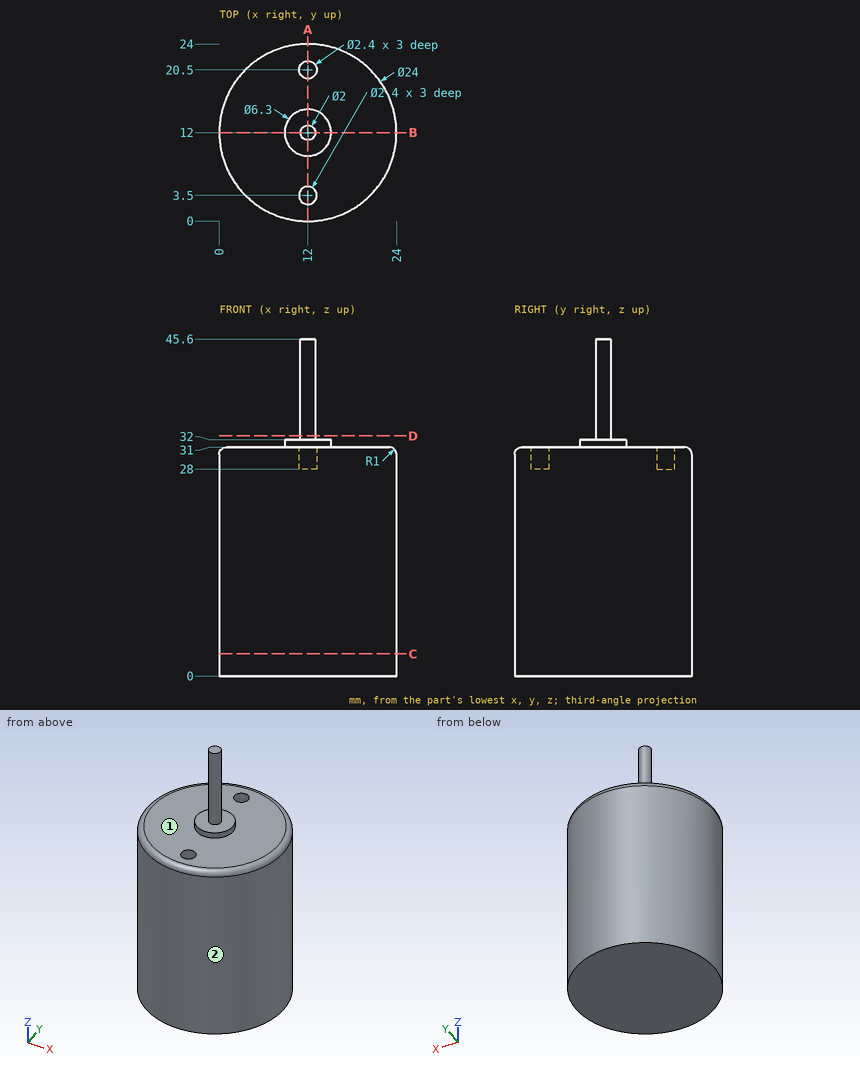
The figure shows three views and two pictorial views of one solid part (mm, origin at its lowest corner). Answer the questions. A direction names the side the tool comes from. Coordinates: 2 decimals unless noted, no trailing zeros. Loops run counter-clockwise (first coordinate to the right, second up) from the corner with the lowest first, then second, coordinate; pieces in that order, holes last.
(1) The part is cut by section D-D (z = 32.5). Determine the outline of the cut face in (x, y), and give its area (3 significant figures).
Solution:
outline: circle Ø2 at (12, 12)
area: 3.14 mm2
(2) The part is cut by section B-B (y = 12). Determine the outline of the cut face in (x, z).
Solution:
outline: (0, 0) - (24, 0) - (24, 30) arc R1 ccw to (23, 31) - (15.15, 31) - (15.15, 32) - (13, 32) - (13, 45.6) - (11, 45.6) - (11, 32) - (8.85, 32) - (8.85, 31) - (1, 31) arc R1 ccw to (0, 30) - close
(3) The part is cut by section C-C (z = 3). Determine the outline of the cut face in (x, y), and give its area (3 significant figures).
Solution:
outline: circle Ø24 at (12, 12)
area: 452 mm2
(4) A tool of negligible diameter and unlimited length cuts with its end or side. For the marked faces 1 and 2, from which of +Z, -Z, +X, -X, +Y, -Y can it reach the whole face along a straight path? Write none if from no direction.
Solution:
face 1: +Z
face 2: +Z, -Z
(5) Flat-ended cylindrical pins translate along their axes: pin 1 Ø4 at (y, z) = (8, 11) entering from +X; pin 2 Ø2 at (y, z) = (4.5, 12) entering from -X; pin 3 Ø1 at (x, y) = (20.5, 17) entering from +Z. Find the tip coordinate at first contact, or state that the pin passes through.
Solution:
pin 1: stops at x = 23.83
pin 2: stops at x = 1.91
pin 3: stops at z = 31
(6) Consider line 1 along Y through (x, z) = (12, 29.7); line 2 along Z through (x, y) = (18, 7.75); line 3 along X through (y, z) = (20.5, 29.5). Determine where each line is inside the solid, lowest interval first.
Solution:
line 1: y = 0 to 2.3, 4.7 to 19.3, 21.7 to 24
line 2: z = 0 to 31
line 3: x = 3.53 to 10.8, 13.2 to 20.47
(7) The part is cut by section A-A (x = 12). Determine the outline of the cut face in (y, z), and give its area (3 significant figures).
Solution:
outline: (0, 0) - (24, 0) - (24, 30) arc R1 ccw to (23, 31) - (21.7, 31) - (21.7, 28) - (19.3, 28) - (19.3, 31) - (15.15, 31) - (15.15, 32) - (13, 32) - (13, 45.6) - (11, 45.6) - (11, 32) - (8.85, 32) - (8.85, 31) - (4.7, 31) - (4.7, 28) - (2.3, 28) - (2.3, 31) - (1, 31) arc R1 ccw to (0, 30) - close
area: 763 mm2
